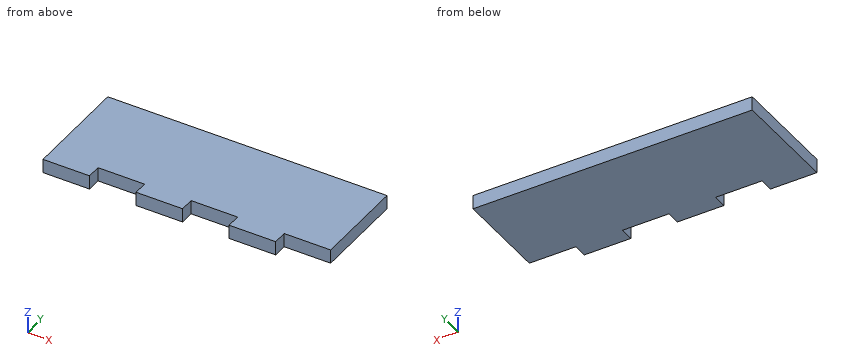
from build123d import *

# Parameters (mm, degrees)
F1_DEPTH = 1.5


with BuildPart() as f1:
    # F0 (on Top) → F1 (new body, symmetric)
    with BuildSketch(Plane.XY):
        Polygon((30, 10), (-30, 10), (-30, -10), (-30, -13), (-20, -13), (-20, -10), (-10, -10), (-10, -13), (0, -13), (0, -10), (10, -10), (10, -13), (20, -13), (20, -10), (30, -10), align=None)
    extrude(amount=F1_DEPTH, both=True)


solid = f1.part
For this review, take the finished solid that the model builds, in its own axes (mm). Round coordinates to 2 decimals unless told otherwise and drop trailing zeros. Order: outer loops, then holes, each group sorted by start corner. A loop starts at its lowest first (then second) coordinate and runs counter-clockwise, first axis right, second up. Notation, with made-up numbers: M 13,-20.5 L 38,-20.5 A9 cw 38,-14.5 Z; hole C 9,35.25 d7. An arc over 180 degrees is marked long. Write each question's results on one line, items separated by ' | '. Start each with the question number.
1. Clearance check with flat-ended pins moving along their axes: pin 1 Ø1.5 at (y, z) = (-11, -0.5) entering from +X; pin 2 Ø0.9 at (x, z) = (-17, 0.5) entering from -Y. State where each tip first meets the part, or that it passes through.
2. Add section B-B (x = 5). State the section outline as (y, z) points.
3. Add section A-A (z = 0.45). State the section outline as (x, y) points.
4. To check wall thickness, follow L1, parallel to X at y = -11.5, z = 0.95; L2, parallel to Y at x = 23.5, z = 1.25. State the ranges of each line that lie inside material, in increasing order. Write a range as [from, to].
Output values:
1) pin 1: x = 20 | pin 2: y = -10
2) outline: M -10,-1.5 L 10,-1.5 L 10,1.5 L -10,1.5 Z
3) outline: M -30,-13 L -20,-13 L -20,-10 L -10,-10 L -10,-13 L 0,-13 L 0,-10 L 10,-10 L 10,-13 L 20,-13 L 20,-10 L 30,-10 L 30,10 L -30,10 Z
4) L1: [-30, -20], [-10, 0], [10, 20] | L2: [-10, 10]
